Source: CAD feature listing. Evaluate the final solid. Frame: model axes, mm. Face numbers are marked on the shaded views. A direction names the side the tool comes from. Coordinates: 2 decimals unless noted, no trailing zeros. Loops run counter-clockwise (first coordinate to the right, second up) from the corner with the lowest first, then second, coordinate; pieces in that order, holes last. Notation, with made-up numbers: (86, 85) - (129, 85) arc R25 ccw to (129, 106) - close; hole circle Ø1 at (43, 63.25). An arc over 180 degrees is marked (long way). Write item = value, one per line. Start each with the question number.
from build123d import *

# Parameters (mm, degrees)
SKETCH1_R           = 5
SKETCH1_R_2         = 0.5
BOSS_EXTRUDE1_DEPTH = 4
SKETCH2_R           = 0.95
CUT_EXTRUDE1_DEPTH  = 2


with BuildPart() as part:
    # Sketch1 → Boss-Extrude1 (new body)
    with BuildSketch(Plane(origin=(0, 0, 0), x_dir=(1, 0, 0), z_dir=(0, 1, 0))):
        Circle(SKETCH1_R)
        with Locations((0, 3.75)):
            Circle(SKETCH1_R_2, mode=Mode.SUBTRACT)
        with Locations((0, -3.75)):
            Circle(SKETCH1_R_2, mode=Mode.SUBTRACT)
    extrude(amount=BOSS_EXTRUDE1_DEPTH)

    # Sketch2 → Cut-Extrude1 (cut)
    with BuildSketch(Plane(origin=(0, 4, 0), x_dir=(1, 0, 0), z_dir=(0, 1, 0))):
        with Locations((0, 3.75)):
            Circle(SKETCH2_R)
        with Locations((0, -3.75)):
            Circle(SKETCH2_R)
    extrude(amount=-CUT_EXTRUDE1_DEPTH, mode=Mode.SUBTRACT)


solid = part.part
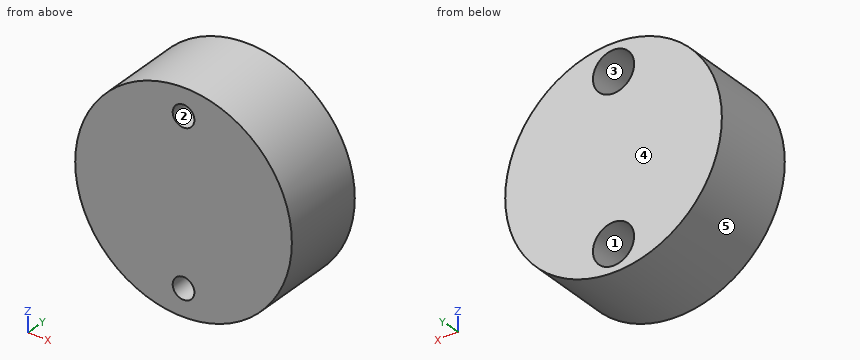
Item 1: Material intervals for L1, parallel to Z at x = 0, y = 3.4; L2, parallel to Z at x = 0.5, y = 3.45; L3, parallel to X at y = 3.35, z = -3, sorted ascending. Write a range as [from, to].
Item 2: First-contact query: pin 1 (1.1 mm diameter, centred on x = 0, z = 3.75, fed in from +Y); pin 2 (2 mm diameter, centred on x = 0, z = -3.75, fed in from -Y); pin 3 (1.5 mm diameter, centred on y = 0.5, z = -2.5, fed in from -X). Flat tips, straight axial feed; report the tip coordinate or a pass-through.
Item 3: Draft query along X for the marked faces 3, 4 and 5. Return one class per face: released by +X, released by -X, zero draft, split by the parting line, or undercut.
Item 4: Cut plane A-A (x = 0). Return the cut outline in (y, z).
Item 5: Cut plane B-B (z = -3.75). Return the cut outline in (x, y), then the cut area to 3 significant figures.
Item 6: Cut plane C-C (y = 2.4). Return the cut outline in (x, z), then the cut area to 3 significant figures.
Item 7: Reachability of the marked faces 1 and 2 from +Z, -Z, +X, -X, +Y, -Y: full face, straight path, thin tool, end or side. Return the list, or none.
Item 8: Cut plane D-D (x = 3). Return the cut outline in (y, z), then the cut area to 3 significant figures.
Responses:
q1.L1 = [-5, -4.7], [-2.8, 2.8], [4.7, 5]
q1.L2 = [-4.97, -4.56], [-2.94, 2.94], [4.56, 4.97]
q1.L3 = [-4, -0.58], [0.58, 4]
q2.pin_1 = 2
q2.pin_2 = 0
q2.pin_3 = -4.68
q3.face_3 = undercut
q3.face_4 = zero draft
q3.face_5 = split by the parting line
q4.outline = (0, -5) - (4, -5) - (4, -4.7) - (2, -4.7) - (2, -4.25) - (0, -4.25) - close; (0, -3.25) - (2, -3.25) - (2, -2.8) - (4, -2.8) - (4, 2.8) - (2, 2.8) - (2, 3.25) - (0, 3.25) - close; (0, 4.25) - (2, 4.25) - (2, 4.7) - (4, 4.7) - (4, 5) - (0, 5) - close
q5.outline = (-3.31, 0) - (-0.5, 0) - (-0.5, 2) - (-0.95, 2) - (-0.95, 4) - (-3.31, 4) - close; (0.5, 0) - (3.31, 0) - (3.31, 4) - (0.95, 4) - (0.95, 2) - (0.5, 2) - close
q5.area = 20.7 mm2
q6.outline = circle Ø10 at (0, 0); hole circle Ø1.9 at (0, -3.75); hole circle Ø1.9 at (0, 3.75)
q6.area = 72.9 mm2
q7.face_1 = +Y
q7.face_2 = +Y, -Y
q8.outline = (0, -4) - (4, -4) - (4, 4) - (0, 4) - close
q8.area = 32.0 mm2
